Source: CAD feature listing. Evaluate the final solid. Frame: model axes, mm. A direction names the side the tool comes from. Give positions to 0.01 mm unless a question says otherwise; leave off trailing zeros. Loops run counter-clockwise (first coordinate to the right, second up) from the corner with the lowest first, then second, coordinate; pieces in that order, holes last. Notation, with made-up numbers: M 16,85 L 64,85 A28 cw 64,109 Z; hole C -13,-25.75 d6. An arc over 180 degrees is marked long. Put each result on its own line as item: value. Start each with the question number.
```python
from build123d import *

# Parameters (mm, degrees)
EXTRUDE_3_DEPTH          = 13
CUT_EXTRUDE_1_DEPTH      = 10
CUT_EXTRUDE_1_DEPTH_BACK = 3.5
SKETCH_5_R               = 0.9
CUT_EXTRUDE_2_DEPTH      = 3.9
SKETCH_7_R               = 4.1
CUT_EXTRUDE_3_DEPTH      = 3
SKETCH_8_R               = 3
CUT_EXTRUDE_4_DEPTH      = 10
CHAMFER_1_SIZE           = 2
FILLET_1_R               = 3


with BuildPart() as part:
    # Эскиз3 → Бобышка-Вытянуть3 (new body)
    with BuildSketch(Plane.XY):
        Polygon((37, -6.101609525), (31, -6.101609525), (31, 35.715183329), (20.718431003, 45.425453097), (-4.040001338, 45.425453097), (-14.040001338, 35.425453097), (-14.040001338, 10.425453097), (-19.540001338, 10.425453097), (-19.457025681, 41.54590709), (-9.338005437, 51.425453097), (-19.457025681, 61.304999103), (-19.540001338, 92.425453097), (-14.040001338, 92.425453097), (-14.040001338, 67.425453097), (-4.040001338, 57.425453097), (20.718431003, 57.425453097), (31, 67.135722864), (31, 108.952515718), (37, 108.952515718), (37, 61.925453097), (25.882237358, 51.425453097), (37, 40.925453097), align=None)
    extrude(amount=EXTRUDE_3_DEPTH)

    # Эскиз4 → Вырез-Вытянуть1 (cut, two sides: drawn at the far end of the back side and taken through both)
    with BuildSketch(Plane(origin=(-19.567659345, 0.052172741, 0), x_dir=(0, 0, 1), z_dir=(-0.9999964455104726, 0.0026662645068428353, 0)).offset(-CUT_EXTRUDE_1_DEPTH_BACK)):
        with BuildLine():
            Line((2.257723781, 10.373317227), (10.742275161, 10.373317227))
            Line((10.742275161, 10.373317227), (9.300003079, 20.36302214))
            ThreePointArc((9.300003079, 20.36302214), (6.5, 23.163025219), (3.699996921, 20.36302214))
            Line((3.699996921, 20.36302214), (2.257723781, 10.373317227))
        make_face()
        with BuildLine():
            Line((10.701924393, 92.093833026), (9.300003079, 82.383612315))
            ThreePointArc((9.300003079, 82.383612315), (6.5, 79.583609236), (3.699996921, 82.383612315))
            Line((3.699996921, 82.383612315), (2.298075607, 92.093833026))
            Line((2.298075607, 92.093833026), (2.298075607, 92.652801429))
            Line((2.298075607, 92.652801429), (10.701924393, 92.652801429))
            Line((10.701924393, 92.652801429), (10.701924393, 92.093833026))
        make_face()
    extrude(amount=CUT_EXTRUDE_1_DEPTH + CUT_EXTRUDE_1_DEPTH_BACK, mode=Mode.SUBTRACT)

    # Эскиз5 → Вырез-Вытянуть2 (cut)
    with BuildSketch(Plane(origin=(-16.067671786, 0.042840815, 0), x_dir=(0, 0, 1), z_dir=(-0.9999964455104726, 0.0026662645068428353, 0))):
        with Locations(Location((6.5, 20.250905412, 0), (0, 0, 270))):
            Circle(SKETCH_5_R)
        with Locations(Location((6.5, 17.200915994, 0), (0, 0, 270))):
            Circle(SKETCH_5_R)
        with Locations(Location((6.5, 14.150926575, 0), (0, 0, 270))):
            Circle(SKETCH_5_R)
        with Locations(Location((6.5, 88.64981885, 0), (0, 0, 90))):
            Circle(SKETCH_5_R)
        with Locations(Location((6.5, 85.599829432, 0), (0, 0, 90))):
            Circle(SKETCH_5_R)
        with Locations(Location((6.5, 82.549840014, 0), (0, 0, 90))):
            Circle(SKETCH_5_R)
    extrude(amount=-CUT_EXTRUDE_2_DEPTH, mode=Mode.SUBTRACT)

    # Эскиз7 → Вырез-Вытянуть3 (cut)
    with BuildSketch(Plane.ZY.offset(-31)):
        with Locations(Location((6.5, 3.89666543, 0), (0, 0, 270))):
            Circle(SKETCH_7_R)
        with Locations(Location((6.5, 98.954240763, 0), (0, 0, 90))):
            Circle(SKETCH_7_R)
    extrude(amount=-CUT_EXTRUDE_3_DEPTH, mode=Mode.SUBTRACT)

    # Эскиз8 → Вырез-Вытянуть4 (cut)
    with BuildSketch(Plane.ZY.offset(-34)):
        with Locations(Location((6.5, 3.89666543, 0), (0, 0, 270))):
            Circle(SKETCH_8_R)
        with Locations((6.5, 98.954240763)):
            Circle(SKETCH_8_R)
    extrude(amount=-CUT_EXTRUDE_4_DEPTH, mode=Mode.SUBTRACT)

    # Фаска1
    chamfer_1_edges = [part.edges().sort_by_distance(p)[0] for p in [
        (25.859215501, 40.570318213, 13),
        (31, 14.806786902, 13),
        (34, -6.101609525, 13),
        (-14.040001338, 22.925453097, 0),
        (37, 17.411921786, 13),
        (-16.790001338, 10.425453097, 0),
        (-19.498513509, 25.985680093, 0),
        (-14.397515559, 46.485680093, 0),
        (-14.397515559, 56.3652261, 0),
        (-19.498513509, 76.8652261, 0),
        (-16.790001338, 92.425453097, 0),
        (-14.040001338, 79.925453097, 0),
        (31.441118679, 46.175453097, 13),
        (-9.040001338, 62.425453097, 0),
        (8.339214833, 57.425453097, 0),
        (25.859215501, 62.28058798, 0),
        (31, 88.044119291, 0),
        (34, 108.952515718, 0),
        (37, 85.438984407, 0),
        (31.441118679, 56.675453097, 0),
        (31.441118679, 46.175453097, 0),
        (31.441118679, 56.675453097, 13),
        (37, 17.411921786, 0),
        (34, -6.101609525, 0),
        (31, 14.806786902, 0),
        (25.859215501, 40.570318213, 0),
        (8.339214833, 45.425453097, 0),
        (-9.040001338, 40.425453097, 0),
        (37, 85.438984407, 13),
        (34, 108.952515718, 13),
        (31, 88.044119291, 13),
        (25.859215501, 62.28058798, 13),
        (-9.040001338, 40.425453097, 13),
        (8.339214833, 57.425453097, 13),
        (-9.040001338, 62.425453097, 13),
        (-14.040001338, 79.925453097, 13),
        (-16.790001338, 92.425453097, 13),
        (-19.498513509, 76.8652261, 13),
        (-14.397515559, 56.3652261, 13),
        (-14.397515559, 46.485680093, 13),
        (-19.498513509, 25.985680093, 13),
        (-16.790001338, 10.425453097, 13),
        (-14.040001338, 22.925453097, 13),
        (8.339214833, 45.425453097, 13),
    ]]
    chamfer(chamfer_1_edges, length=CHAMFER_1_SIZE)

    # Скругление1
    # the kernel refuses this fillet: 3 mm, written as the material it takes off along each edge
    with BuildSketch(Plane(origin=(31, 108.952515718, -5.5), x_dir=(1, 0, 0), z_dir=(0, 0, 1)), Plane(origin=(37, 108.952515718, -5.5), x_dir=(0, -1, 0), z_dir=(0, 0, 1)), Plane(origin=(37, -6.101609525, -5.5), x_dir=(-1, 0, 0), z_dir=(0, 0, 1))) as fillet_1_piece_1:
        with BuildLine():
            CenterArc((FILLET_1_R, -FILLET_1_R), FILLET_1_R, 90, 90)
            Line((0, -FILLET_1_R), (0, 0))
            Line((0, 0), (FILLET_1_R, 0))
        make_face()
    extrude(amount=24, mode=Mode.SUBTRACT)
    with BuildSketch(Plane(origin=(27.893398282, 108.952515718, 2), x_dir=(0, -0.7071067811865495, -0.7071067811865456), z_dir=(1, 0, 0)), Plane(origin=(40.106601718, -6.101609525, 11), x_dir=(0, 0, -1), z_dir=(-1, 0, 0))) as fillet_1_piece_2:
        with BuildLine():
            CenterArc((FILLET_1_R * 0.414213562373, -FILLET_1_R), FILLET_1_R, 90, 45)
            Line((-FILLET_1_R * 0.292893218813, -FILLET_1_R * 0.292893218813), (0, 0))
            Line((0, 0), (FILLET_1_R * 0.414213562373, 0))
        make_face()
    extrude(amount=12.213203436, mode=Mode.SUBTRACT)
    with BuildSketch(Plane(origin=(27.893398282, 108.952515718, 11), x_dir=(0, -0.7071067811865481, 0.7071067811865467), z_dir=(1, 0, 0)), Plane(origin=(40.106601718, -6.101609525, 2), x_dir=(0, 0, 1), z_dir=(-1, 0, 0))) as fillet_1_piece_3:
        with BuildLine():
            CenterArc((FILLET_1_R * 0.414213562373, FILLET_1_R), FILLET_1_R, 225, 45)
            Line((-FILLET_1_R * 0.292893218813, FILLET_1_R * 0.292893218813), (0, 0))
            Line((0, 0), (FILLET_1_R * 0.414213562373, 0))
        make_face()
    extrude(amount=12.213203436, mode=Mode.SUBTRACT)
    with BuildSketch(Plane(origin=(31, -6.101609525, -5.5), x_dir=(1, 0, 0), z_dir=(0, 0, 1))) as fillet_1_piece_4:
        with BuildLine():
            CenterArc((FILLET_1_R, FILLET_1_R), FILLET_1_R, 180, 90)
            Line((0, FILLET_1_R), (0, 0))
            Line((0, 0), (FILLET_1_R, 0))
        make_face()
    extrude(amount=24, mode=Mode.SUBTRACT)


solid = part.part
```
1. Section A-A, the plane y = 59.5. Output: boundary loops of the cut face in (x, z), plus the area to 3 significant figures.
2. Section C-C, the plane x = -2.5. Output: boundary loops of the cut face in (y, z).
3. Set-up query: faces 1 (the face through (31.52, 56.75, 6.44)), 2 (the face through (-15, 92.425, 6)), 3 (the face through (-13.057, 46.417, 11.986)), 4 (the face through (26.641, 41.188, 11.986)). Return all of +Z, -Z, +X, -X, +Y, -Y with unobstructed straight access to the full face (end or side cutting, diameter ignored); none if empty.
4. Contact query for flat-ended pins moving along their axis: pin 1 (6 mm diameter, centred on x = -6.5, z = 2.5, fed in from +Y); pin 2 (10 mm diameter, centred on x = 14.5, y = 43.5, fed in from +Z); pin 3 (7 mm diameter, centred on x = 7, z = 6, fed in from -Y); pin 4 (6 mm diameter, centred on x = -18, z = 8.5, fed in from +Y). Output: stop coordinate, or through.
5. Section B-B, the plane x = -12. Output: boundary loops of the cut face in (y, z), plus the area to 3 significant figures.
6. Pull-direction query (X, two-part tool) for faces 5 (the face through (-16.829, 91.662, 11.764)), 6 (the face through (-8.97, 40.495, 6.437)), 7 (the face through (29.906, 46.269, 1.014)); classes: released by +X, released by -X, zero draft, split by the parting line, or undercut.
7. Ray query, line 1 (X direction, y = 30, z = 2.75); line 2 (X direction, y = 20, z = 8); line 3 (X direction, y = 1, z = 7.5). Return the intervals inside material, ascending.
Results found:
1. outline: M -17.61,2 L -14.75,0 L -8.94,0 L -6.11,2 L -6.11,11 L -8.94,13 L -14.75,13 L -17.61,11 Z; M 22.92,2 L 25.83,0 L 31.52,0 L 34.43,2 L 34.43,11 L 31.52,13 L 25.83,13 L 22.92,11 Z
1. area: 276 mm²
2. outline: M 45.43,2 L 47.43,0 L 55.43,0 L 57.43,2 L 57.43,11 L 55.43,13 L 47.43,13 L 45.43,11 Z
3. face 1: +Z, -Z, +X
3. face 2: +Z, -Z, -X, +Y
3. face 3: +Z, -X
3. face 4: +Z, -Y
4. pin 1: y = 62.89
4. pin 2: z = 13
4. pin 3: y = 45.43
4. pin 4: y = 92.43
5. outline: M 37.47,2 L 40.29,0 L 46.03,0 L 48.83,2 L 48.83,11 L 46.03,13 L 40.29,13 L 37.47,11 Z; M 54.02,2 L 56.82,0 L 62.56,0 L 65.39,2 L 65.39,11 L 62.56,13 L 56.82,13 L 54.02,11 Z
5. area: 273 mm²
6. face 5: zero draft
6. face 6: undercut
6. face 7: released by +X
7. line 1: -19.49 to -14.04, 31 to 37
7. line 2: -16.01 to -14.04, 31 to 37
7. line 3: 34 to 37
